from build123d import *

# Parameters (mm, degrees)
SKETCH1_W           = 5.334
SKETCH1_H           = 33.401
BOSS_EXTRUDE1_DEPTH = 5.461
SKETCH2_W           = 19.05
SKETCH2_H           = 5.461
BOSS_EXTRUDE2_DEPTH = 5.461


with BuildPart() as part:
    # Sketch1 → Boss-Extrude1 (new body)
    with BuildSketch(Plane.XY):
        Polygon((26.289, 32.5755), (-26.289, 32.5755), (-26.289, 16.7005), (-20.828, 16.7005), (-20.828, -16.7005), (-26.289, -16.7005), (-26.289, -32.5755), (26.289, -32.5755), (26.289, -16.7005), (26.289, 16.7005), align=None)
        with Locations((28.956, 0)):
            Rectangle(SKETCH1_W, SKETCH1_H)
    extrude(amount=BOSS_EXTRUDE1_DEPTH)

    # Sketch2 → Boss-Extrude2 (add)
    with BuildSketch(Plane.XY.offset(5.461)):
        with Locations((11.9634, 35.306)):
            Rectangle(SKETCH2_W, SKETCH2_H)
        with Locations((11.9634, -35.306)):
            Rectangle(SKETCH2_W, SKETCH2_H)
    extrude(amount=-BOSS_EXTRUDE2_DEPTH)


solid = part.part
Geometry: final body of the model. Coordinates: model frame, mm. A direction names the side the tool comes from. Coordinates: 2 decimals unless noted, no trailing zeros. Loops run counter-clockwise (first coordinate to the right, second up) from the corner with the lowest first, then second, coordinate; pieces in that order, holes last. Notation, with made-up numbers: M 66.25,86 L 86.25,86 A18 ccw 86.25,119 Z; hole C -35,-6.5 d3. An arc over 180 degrees is marked long. One line per item, written item: value. Start each with the question number.
1) Material intervals for L1, parallel to Y at x = -8.5, z = 0.85; L2, parallel to X at y = -29.5, z = 2.8; L3, parallel to Y at x = 28.5, z = 3.8, sorted ascending. Write a range as from..to.
2) Pin query (flat end, axial travel): P1, Ø2.5, axis at x = -22.5, z = 3, coming from the +Y side; P2, Ø1.6, axis at y = 35, z = 2, coming from the -X side; P3, Ø2.5, axis at y = 28, z = 3, coming from the +X side. Return the tip coordinate at first contact, or that it passes through.
3) Reachability of faces 4 (the flat face through (26.289, 25, 3)), 5 (the flat face through (2.438, -35, 3)), 6 (the flat face through (24, -32.575, 3)) from +Z, -Z, +X, -X, +Y, -Y: full face, straight path, thin tool, end or side. Return the list, or none.
4) Cut plane B-B (z = 2.65). Return loops of the section in (x, y).
5) Cut plane D-D (x = -13.5). Return loops of the section in (y, z).
6) Draft query along Y for faces 1 (the flat face through (-24, 16.7, 3)), 2 (the flat face through (-12, 32.575, 3)), 3 (the flat face through (12, -38.036, 3)). Return one class per face: released by +Y, released by -Y, zero draft, split by the parting line, or undercut.
7) Cut plane C-C (y = -2). Return loops of the section in (x, z).
8) Cut plane A-A (x = -22). Return loops of the section in (y, z).
Evaluation:
1. L1: -32.58..32.58
1. L2: -26.29..26.29
1. L3: -16.7..16.7
2. P1: y = 32.58
2. P2: x = 2.44
2. P3: x = 26.29
3. face 4: +Z, -Z, +X, +Y
3. face 5: +Z, -Z, -X, -Y
3. face 6: +Z, -Z, +X, -Y
4. outline: M -26.29,-32.58 L 2.44,-32.58 L 2.44,-38.04 L 21.49,-38.04 L 21.49,-32.58 L 26.29,-32.58 L 26.29,-16.7 L 31.62,-16.7 L 31.62,16.7 L 26.29,16.7 L 26.29,32.58 L 21.49,32.58 L 21.49,38.04 L 2.44,38.04 L 2.44,32.58 L -26.29,32.58 L -26.29,16.7 L -20.83,16.7 L -20.83,-16.7 L -26.29,-16.7 Z
5. outline: M -32.58,0 L 32.58,0 L 32.58,5.46 L -32.58,5.46 Z
6. face 1: undercut
6. face 2: released by +Y
6. face 3: released by -Y
7. outline: M -20.83,0 L 31.62,0 L 31.62,5.46 L -20.83,5.46 Z
8. outline: M -32.58,0 L -16.7,0 L -16.7,5.46 L -32.58,5.46 Z; M 16.7,0 L 32.58,0 L 32.58,5.46 L 16.7,5.46 Z
